Part model, mm, in its own coordinate system. A direction names the side the tool comes from. Round coordinates to 2 decimals unless told otherwise and drop trailing zeros. Order: outer loops, then holes, each group sorted by start corner. A loop starts at its lowest first (then second) coordinate and runs counter-clockwise, first axis right, second up. Notation, with made-up numbers: (32, -28) -> (50, -28) arc R16 cw to (50, -11) -> close; hole circle Ø3 at (2.25, 52.25). An arc over 180 degrees is marked (long way). Use CSV: the item, a comma, the result in double quotes.
```python
from build123d import *

# Parameters (mm, degrees)
F0_R      = 24
F1_DEPTH  = 35
F2_START  = 1
F0_R_2    = 22
F2_DEPTH  = 2
F3_START  = -27
F2_FACE_R = 24
F3_DEPTH  = 15.1
F4_R      = 22
F5_DEPTH  = 40.5


with BuildPart() as f1:
    # F0 (on Front) → F1 (new body)
    with BuildSketch(Plane.XZ):
        with BuildLine():
            ThreePointArc((-25.9229627936, 2), (-26, 0), (-25.9229627936, -2))
            ThreePointArc((-25.9229627936, -2), (0, -26), (25.9229627936, -2))
            ThreePointArc((25.9229627936, -2), (26, 0), (25.9229627936, 2))
            ThreePointArc((25.9229627936, 2), (0, 26), (-25.9229627936, 2))
        make_face()
        Circle(F0_R, mode=Mode.SUBTRACT)
    extrude(amount=F1_DEPTH)

    # F0 (on Front) → F2 (join)
    with BuildSketch(Plane.XZ.offset(F2_START)):
        Circle(F0_R)
        Circle(F0_R_2, mode=Mode.SUBTRACT)
        Circle(F0_R_2)
    extrude(amount=F2_DEPTH)

    # F2_face (on face) → F3 (join)
    with BuildSketch(Plane(origin=(0, -1, 0), x_dir=(1, 0, 0), z_dir=(0, 1, 0)).offset(F3_START)):
        Circle(F2_FACE_R)
    extrude(amount=-F3_DEPTH)

    # F4 (on face) → F5 (cut)
    with BuildSketch(Plane.XZ.offset(43.1)):
        Circle(F4_R)
    extrude(amount=-F5_DEPTH, mode=Mode.SUBTRACT)


solid = f1.part
```
(1) Probe probe 1 along Y at (x, z) = (19, -12.5); probe 2 along Y at (x, z) = (-8.5, 2); probe 3 along Z at (x, y) = (11.5, -11). List the from-to ranges inside material, lowest first. Write a range as [from, to].
Reply:
probe 1,"[-43.1, -28], [-3, -1]"
probe 2,"[-2.6, -1]"
probe 3,"[-23.32, -21.07], [21.07, 23.32]"
(2) Cut at C-C, the plane x = 0. Give the cut face in (y, z), then the cut area to 3 significant figures.
Reply:
outline,"(-43.1, -24) -> (-35, -24) -> (-35, -26) -> (0, -26) -> (0, -24) -> (-1, -24) -> (-1, 24) -> (0, 24) -> (0, 26) -> (-35, 26) -> (-35, 24) -> (-43.1, 24) -> (-43.1, 22) -> (-28, 22) -> (-28, 24) -> (-3, 24) -> (-3, 22) -> (-2.6, 22) -> (-2.6, -22) -> (-3, -22) -> (-3, -24) -> (-28, -24) -> (-28, -22) -> (-43.1, -22) -> close"
area,"279 mm2"
(3) Which spindle directions (+Z, -Z, +X, -X, +Y, -Y) get a long thin tool onto all of the face, cutting with end or side? Do faces 4 (the face through (0, -2.6, 0)), 5 (the face through (7, -3, -21.2)), 6 (the face through (-23.977, -0.493, 1.055)). Say none if no direction does.
Reply:
face 4,"-Y"
face 5,"none"
face 6,"+Y"
(4) Cut at B-B, the plane y = -6.5. Give the cut face in (x, z).
Reply:
outline,"circle Ø52 at (0, 0); hole circle Ø48 at (0, 0)"
(5) Drop flat-ended pins along their axis: P1, Ø1.5, axis at y = -28.5, z = 13, coming from the +X side; P2, Ø3, axis at y = -15, z = 17.5, coming from the +X side; P3, Ø14.5, axis at x = -11, z = 9, coming from the +Y side; P4, Ø2, axis at y = -29.5, z = -0.5, coming from the -X side. Give the stop position or say it passes through.
Reply:
P1,"x = 22.93"
P2,"x = 20.49"
P3,"y = -1"
P4,"x = -26"
(6) Pull direction Z, two halves, no side cores. Call faces 1 (the face through (8, 0, -23)), 2 (the face through (-23.977, -38.993, -1.055)), 3 (the face through (-4.769, -2.803, -21.477)): released by +Z, released by -Z, zero draft, split by the parting line, or undercut.
Reply:
face 1,"zero draft"
face 2,"split by the parting line"
face 3,"undercut"
(7) Cut at A-A, the plane z = 0. Give the cut face in (x, y).
Reply:
outline,"(-26, -35) -> (-24, -35) -> (-24, -43.1) -> (-22, -43.1) -> (-22, -28) -> (-24, -28) -> (-24, -3) -> (-22, -3) -> (-22, -2.6) -> (22, -2.6) -> (22, -3) -> (24, -3) -> (24, -28) -> (22, -28) -> (22, -43.1) -> (24, -43.1) -> (24, -35) -> (26, -35) -> (26, 0) -> (24, 0) -> (24, -1) -> (-24, -1) -> (-24, 0) -> (-26, 0) -> close"
